Input: dimensioned drawing with shaded views. Units: mm. Origin: part minimum x, y, z. Coordinates: 2 decimals unless noted, no trailing zeros. Loops run counter-clockwise (first coordinate to the right, second up) from the corner with the lowest first, then second, coordinate; pieces in that order, holes last.
Item 1: Section A-A on x = 17.78. Return loops of the section in (y, z), and give its area (3 significant figures).
Item 2: Section C-C on x = 10. Return loops of the section in (y, z).
Item 3: Contact query for flat-ended pins moving along their axis: P1, Ø10, axis at x = 13, y = 10.5, coming from the -Z side; P2, Ø1.6, axis at x = 10.5, z = 2.5, coming from the -Y side; P3, Ø5, axis at x = 2.286, y = 17.78, coming from the +Z side; P4, Ø1, axis at y = 18, z = 2.5, coming from the +X side. Output: stop coordinate, or through.
Item 4: Section D-D on z = 0.9. Return loops of the section in (x, y).
Item 5: Ray query, line 1 along Y through (x, z) = (17.78, 0.5); line 2 along Y through (x, z) = (17.25, 0.85); line 3 along Z through (x, y) = (7.25, 17.5). Return the intervals inside material, ascending.
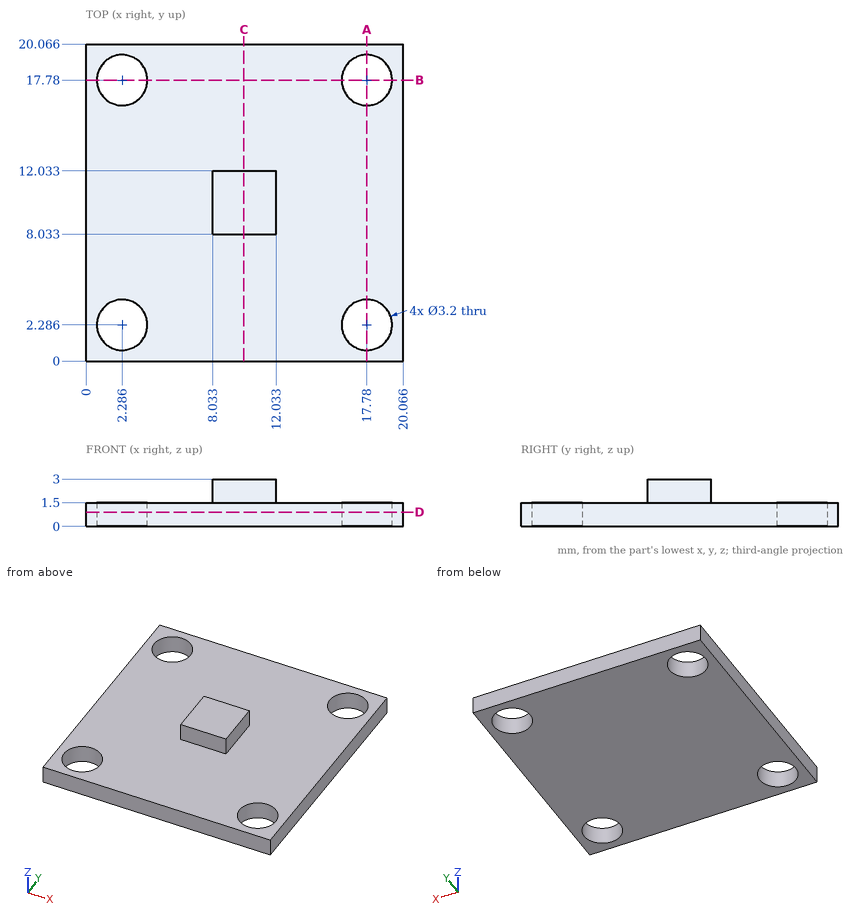
Results found:
1. outline: (0, 0) - (0.69, 0) - (0.69, 1.5) - (0, 1.5) - close; (3.89, 0) - (16.18, 0) - (16.18, 1.5) - (3.89, 1.5) - close; (19.38, 0) - (20.07, 0) - (20.07, 1.5) - (19.38, 1.5) - close
1. area: 20.5 mm2
2. outline: (0, 0) - (20.07, 0) - (20.07, 1.5) - (12.03, 1.5) - (12.03, 3) - (8.03, 3) - (8.03, 1.5) - (0, 1.5) - close
3. P1: stops at z = 0
3. P2: stops at y = 8.03
3. P3: stops at z = 1.5
3. P4: passes through
4. outline: (0, 0) - (20.07, 0) - (20.07, 20.07) - (0, 20.07) - close; hole circle Ø3.2 at (2.29, 2.29); hole circle Ø3.2 at (2.29, 17.78); hole circle Ø3.2 at (17.78, 2.29); hole circle Ø3.2 at (17.78, 17.78)
5. line 1: y = 0 to 0.69, 3.89 to 16.18, 19.38 to 20.07
5. line 2: y = 0 to 0.78, 3.8 to 16.27, 19.29 to 20.07
5. line 3: z = 0 to 1.5
